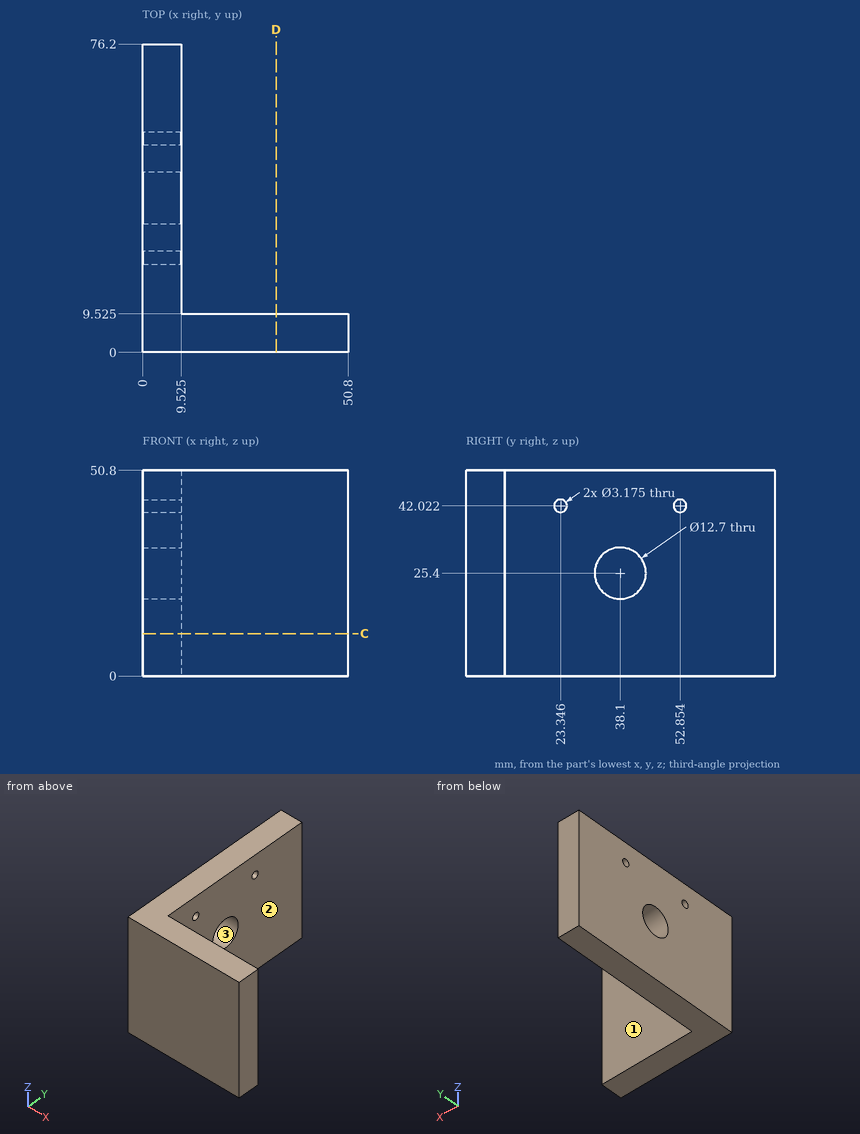
For this review, use the dimensioned drawing (mm, ordinates from the lowest corner) and the shaded views. Coordinates: 2 decimals unless noted, no trailing zeros. Loops run counter-clockwise (first coordinate to the right, second up) from the corner with the lowest first, then second, coordinate; pieces in that order, holes last. Notation, with made-up numbers: (62, 60) -> (82, 60) arc R27 ccw to (82, 97) -> close; hole circle Ø4 at (9.25, 82). An arc over 180 degrees is marked (long way). Write each question's results on one line, items separated by ' | '.
Q1. Mouldability with a two-part tool opening along Y and no side actions: class the marked faces 1, 2 and 3 as +Y half, -Y half, draft (parallel to the pull), parting line (faces both ways), or undercut.
Taken from the geometry:
face 1: +Y half | face 2: draft | face 3: undercut
Q2. Add section D-D, the plane x = 33. State the section outline as (y, z) points (1 decimal).
Taken from the geometry:
outline: (0, 0) -> (9.5, 0) -> (9.5, 50.8) -> (0, 50.8) -> close
Q3. Add section C-C, the plane z = 10.5. State the section outline as (x, y) points (1 decimal).
Taken from the geometry:
outline: (0, 0) -> (50.8, 0) -> (50.8, 9.5) -> (9.5, 9.5) -> (9.5, 76.2) -> (0, 76.2) -> close
Q4. For pin 1 Ø1.9 at (y, z) = (52.85, 42.02) entering from +X (3 decimals); pin 2 Ø5 at (x, z) = (15, 14) entering from +Y (1 decimal); pin 3 Ø15 at (y, z) = (55.5, 29) entering from +X (1 decimal), all flat-tipped, find the tip position at first contact; note any pin that passes through.
Taken from the geometry:
pin 1: through | pin 2: y = 9.5 | pin 3: x = 9.5
Q5. To check wall thickness, follow line 1 along Y through (x, z) = (6.5, 42); line 2 along X through (y, z) = (71, 20) (1 decimal). State the ranges of each line that lie inside material, in increasing order. Write a range as [from, to].
Taken from the geometry:
line 1: [0, 21.76], [24.93, 51.27], [54.44, 76.2] | line 2: [0, 9.5]
